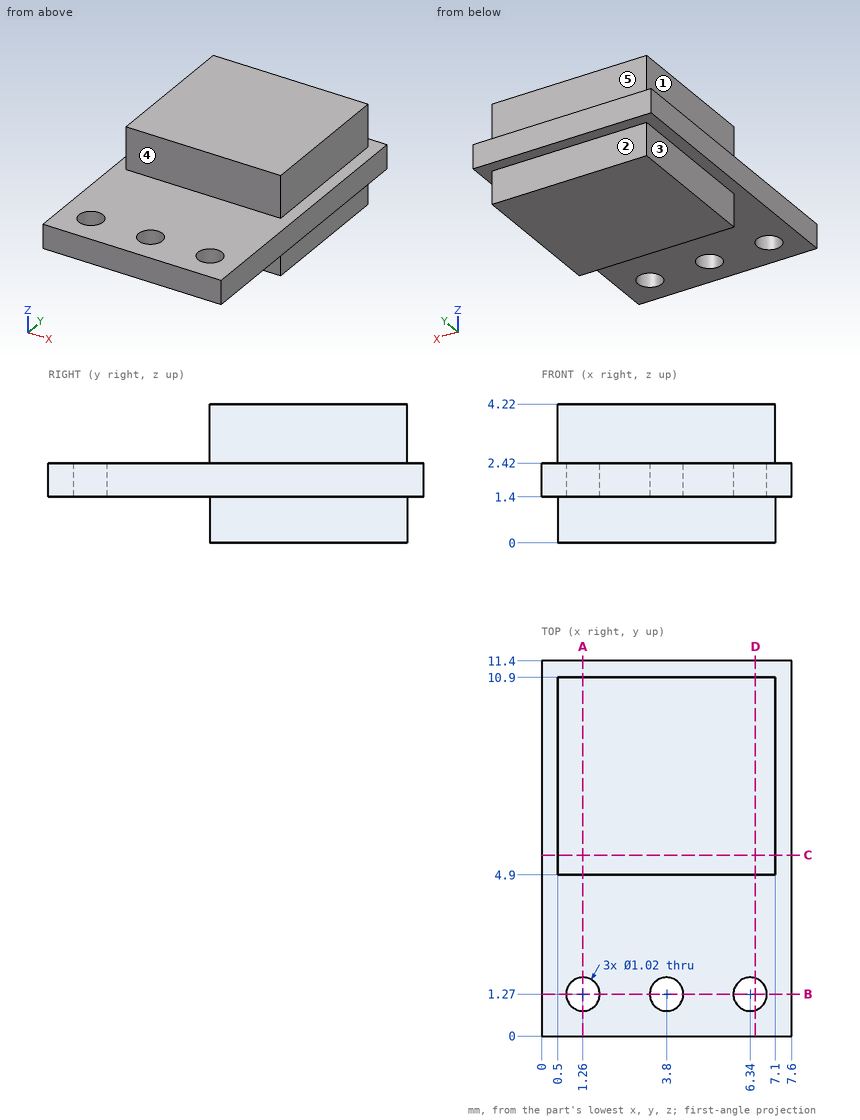
The figure shows three views and two pictorial views of one solid part (mm, origin at its lowest corner). Answer the questions. A direction names the side the tool comes from. Give positions to 0.01 mm unless a question says otherwise; leave off trailing zeros. Write each loop counter-clockwise with the first axis right and the second up, starting at its lowest first coordinate (ties: lowest second). Pieces come first, ordered by that corner, then holes. Notation, with made-up numbers: (-10.5, 61) -> (-3.5, 61) arc R13 ccw to (-3.5, 77) -> close; hole circle Ø1 at (62.25, -11.75). An arc over 180 degrees is marked (long way). Use one line per item in the form item = value.
1) Section C-C on y = 5.5 is taken. Write down the section's boundary in (x, z), plus the area to 3 significant figures.
Result:
outline = (0, 1.4) -> (0.5, 1.4) -> (0.5, 0) -> (7.1, 0) -> (7.1, 1.4) -> (7.6, 1.4) -> (7.6, 2.42) -> (7.1, 2.42) -> (7.1, 4.22) -> (0.5, 4.22) -> (0.5, 2.42) -> (0, 2.42) -> close
area = 28.9 mm²
2) Section D-D on x = 6.5 is taken. Write down the section's boundary in (y, z), plus the area to 3 significant figures.
Result:
outline = (0, 1.4) -> (0.79, 1.4) -> (0.79, 2.42) -> (0, 2.42) -> close; (1.75, 1.4) -> (4.9, 1.4) -> (4.9, 0) -> (10.9, 0) -> (10.9, 1.4) -> (11.4, 1.4) -> (11.4, 2.42) -> (10.9, 2.42) -> (10.9, 4.22) -> (4.9, 4.22) -> (4.9, 2.42) -> (1.75, 2.42) -> close
area = 29.8 mm²
3) Section A-A on x = 1.26 is taken. Write down the section's boundary in (y, z), plus the area to 3 significant figures.
Result:
outline = (0, 1.4) -> (0.76, 1.4) -> (0.76, 2.42) -> (0, 2.42) -> close; (1.78, 1.4) -> (4.9, 1.4) -> (4.9, 0) -> (10.9, 0) -> (10.9, 1.4) -> (11.4, 1.4) -> (11.4, 2.42) -> (10.9, 2.42) -> (10.9, 4.22) -> (4.9, 4.22) -> (4.9, 2.42) -> (1.78, 2.42) -> close
area = 29.8 mm²
4) Each of these flat-tipped pins is pushed along its axis until it touches: P1, Ø1.6, axis at x = 3.8, y = 1.27, coming from the -Z side; P2, Ø0.5, axis at x = 3.5, z = 3.5, coming from the -Y side; P3, Ø1.4, axis at x = 2.5, z = 3.5, coming from the +Y side. Where does it stop, or does it pass through?
Result:
P1 = 1.4
P2 = 4.9
P3 = 10.9
5) A tool of negligible diameter and unlimited length cuts with its end or side. For the marked faces 1, 2, 3, 4 and 5, from which of +Z, -Z, +X, -X, +Y, -Y can it reach the whole face along a straight path? Write none if from no direction.
Result:
face_1 = +Z, -X, +Y, -Y
face_2 = -Z, +X, -X, +Y
face_3 = -Z, -X, +Y, -Y
face_4 = +Z, +X, -X, -Y
face_5 = +Z, +X, -X, +Y
6) Section B-B on y = 1.27 is taken. Write down the section's boundary in (x, z), plus the area to 3 significant figures.
Result:
outline = (0, 1.4) -> (0.75, 1.4) -> (0.75, 2.42) -> (0, 2.42) -> close; (1.77, 1.4) -> (3.29, 1.4) -> (3.29, 2.42) -> (1.77, 2.42) -> close; (4.31, 1.4) -> (5.83, 1.4) -> (5.83, 2.42) -> (4.31, 2.42) -> close; (6.85, 1.4) -> (7.6, 1.4) -> (7.6, 2.42) -> (6.85, 2.42) -> close
area = 4.63 mm²
7) Straight lines are drawn through the part: probe 1 along Y at (x, z) = (3.8, 1.7); probe 2 along Y at (x, z) = (2.75, 1); probe 3 along Z at (x, y) = (1.5, 2.5). For each, find the intervals that lie inside material, in ascending order.
Result:
probe_1 = 0 to 0.76, 1.78 to 11.4
probe_2 = 4.9 to 10.9
probe_3 = 1.4 to 2.42
